from build123d import *

# Parameters (mm, degrees)
SKETCH1_R           = 1.5
BOSS_EXTRUDE1_DEPTH = 3
SKETCH2_W           = 6
SKETCH2_H           = 5
SKETCH2_H_2         = 2
BOSS_EXTRUDE2_DEPTH = 26
CUT_EXTRUDE1_REACH  = 34.939
SKETCH3_R           = 1.575
FILLET1_R           = 0.5


with BuildPart() as part:
    # Sketch1 → Boss-Extrude1 (new body)
    with BuildSketch(Plane(origin=(0, 0, 0), x_dir=(1, 0, 0), z_dir=(0, 1, 0))):
        Polygon((-10, 4.075667656), (10, 4.075667656), (10, -0.924332344), (3, -0.924332344), (3, -7.924332344), (-3, -7.924332344), (-3, -0.924332344), (-10, -0.924332344), align=None)
        with Locations(Location((7.5, 1.575667656, 0), (0, 0, 270))):
            Circle(SKETCH1_R, mode=Mode.SUBTRACT)
        with Locations(Location((-7.5, 1.575667656, 0), (0, 0, 270))):
            Circle(SKETCH1_R, mode=Mode.SUBTRACT)
    extrude(amount=BOSS_EXTRUDE1_DEPTH)

    # Sketch2 → Boss-Extrude2 (add)
    with BuildSketch(Plane(origin=(0, 3, 0), x_dir=(1, 0, 0), z_dir=(0, 1, 0))):
        with Locations((0, 1.575667656)):
            Rectangle(SKETCH2_W, SKETCH2_H)
        with Locations((0, -6.924332344)):
            Rectangle(SKETCH2_W, SKETCH2_H_2)
    extrude(amount=BOSS_EXTRUDE2_DEPTH)

    # Cut-Extrude1: up to this face of the body (flat: up to its plane)
    cut_extrude1_end = Plane(part.part.faces().sort_by_distance((0, 14.5, 7.924332344))[0])
    # Sketch3 → Cut-Extrude1 (cut, up to the picked face)
    with BuildSketch(Plane(origin=(0, 0, -4.075667656), x_dir=(-1, 0, 0), z_dir=(0, 0, -1)), mode=Mode.PRIVATE) as cut_extrude1_sk1:
        with Locations((0, 26.75)):
            Circle(SKETCH3_R)
    cut_extrude1_tool1 = split(extrude(cut_extrude1_sk1.sketch, amount=-CUT_EXTRUDE1_REACH, mode=Mode.PRIVATE), bisect_by=cut_extrude1_end, keep=Keep.BOTH, mode=Mode.PRIVATE)
    add(cut_extrude1_tool1.solids().sort_by(Axis((0, 26.75, -4.075668), (0, 0, 1)))[0], mode=Mode.SUBTRACT)

    # Fillet1
    fillet1_edges = [part.edges().sort_by_distance(p)[0] for p in [
        (1.575, 26.75, 0.924332344),
        (1.575, 26.75, 5.924332344),
        (1.575, 26.75, -4.075667656),
        (1.575, 26.75, 7.924332344),
    ]]
    fillet(fillet1_edges, radius=FILLET1_R)


solid = part.part
CAD build for the part. Positions are in the model's coordinates, mm. A direction names the side the tool comes from. Give positions to 0.01 mm unless a question says otherwise; leave off trailing zeros. Write each loop counter-clockwise with the first axis right and the second up, starting at its lowest first coordinate (ties: lowest second). Pieces come first, ordered by that corner, then holes. Notation, with made-up numbers: (25, -11) - (44, -11) arc R34 cw to (44, 24) - close; hole circle Ø5 at (-16, -23). An arc over 180 degrees is marked (long way). Answer as CSV lines item,"result".
Q1. Flat gauge pins, fed straight in: pin 1 Ø4 at (x, z) = (1, 3.5) entering from +Y; pin 2 Ø2.5 at (x, z) = (-7.5, -1.58) entering from +Y; pin 3 Ø2.5 at (x, y) = (5, 1) entering from +Z; pin 4 Ø3.5 at (x, y) = (0, 26.75) entering from +Z. Where does each tip first touch, or does it go through?
Result set:
pin 1,"y = 3"
pin 2,"through"
pin 3,"z = 0.92"
pin 4,"z = 7.8"
Q2. Pull direction Z, two halves, no side cores. Call faces 6 (the face through (6.036, 1.479, -1.901)), 7 (the face through (7, 1, 0.924)), 8 (the face through (3, 11, 7)): released by +Z, released by -Z, zero draft, split by the parting line, or undercut.
Result set:
face 6,"undercut"
face 7,"released by +Z"
face 8,"zero draft"
Q3. Band-saw the part on D-D (y = 12.75). Give the cut face in (x, z).
Result set:
outline,"(-3, -4.08) - (3, -4.08) - (3, 0.92) - (-3, 0.92) - close; (-3, 5.92) - (3, 5.92) - (3, 7.92) - (-3, 7.92) - close"
Q4. Band-saw the part on B-B (x = 0). Give the cut face in (y, z) (3 decimals).
Result set:
outline,"(0, -4.076) - (24.675, -4.076) arc R0.5 ccw to (25.175, -3.576) - (25.175, 0.424) arc R0.5 ccw to (24.675, 0.924) - (3, 0.924) - (3, 5.924) - (24.675, 5.924) arc R0.5 ccw to (25.175, 6.424) - (25.175, 7.424) arc R0.5 ccw to (24.675, 7.924) - (0, 7.924) - close; (28.325, -3.576) arc R0.5 ccw to (28.825, -4.076) - (29, -4.076) - (29, 0.924) - (28.825, 0.924) arc R0.5 ccw to (28.325, 0.424) - close; (28.325, 6.424) arc R0.5 ccw to (28.825, 5.924) - (29, 5.924) - (29, 7.924) - (28.825, 7.924) arc R0.5 ccw to (28.325, 7.424) - close"
Q5. Drill centre lines: line 1 (Y direction, x = 0, z = -1.15) (3 decimals); line 2 (X direction, y = 8.75, z = 7.5); line 3 (Y direction, x = 2, z = 4.75). Where is each one in solid material? Low to high. Write a range as from..to.
Result set:
line 1,"0..25.175, 28.325..29"
line 2,"-3..3"
line 3,"0..3"
Q6. Band-saw the part on A-A (x = 7.5). Give the cut face in (y, z), and give its area (3 significant figures).
Result set:
outline,"(0, -4.08) - (3, -4.08) - (3, -3.08) - (0, -3.08) - close; (0, -0.08) - (3, -0.08) - (3, 0.92) - (0, 0.92) - close"
area,"6.00 mm²"
Q7. Band-saw the part on C-C (y = 26.75). Give the cut face in (x, z) (3 decimals), and give its area (3 significant figures).
Result set:
outline,"(-3, -4.076) - (-2.075, -4.076) arc R0.5 ccw to (-1.575, -3.576) - (-1.575, 0.424) arc R0.5 ccw to (-2.075, 0.924) - (-3, 0.924) - close; (-3, 5.924) - (-2.075, 5.924) arc R0.5 ccw to (-1.575, 6.424) - (-1.575, 7.424) arc R0.5 ccw to (-2.075, 7.924) - (-3, 7.924) - close; (1.575, -3.576) arc R0.5 ccw to (2.075, -4.076) - (3, -4.076) - (3, 0.924) - (2.075, 0.924) arc R0.5 ccw to (1.575, 0.424) - close; (1.575, 6.424) arc R0.5 ccw to (2.075, 5.924) - (3, 5.924) - (3, 7.924) - (2.075, 7.924) arc R0.5 ccw to (1.575, 7.424) - close"
area,"19.5 mm²"
Q8. 3-axis set-ups, long thin cutter, end or side, ignore diameter. For faces 1 (the face through (0, 16, 5.924)), 2 (the face through (0, 11, -4.076)), 3 (the face through (5.8, 3, -1.6)), 4 (the face through (-3, 11, 7)), 5 (the face through (-3, 16, -2)): which of +Z, -Z, +X, -X, +Y, -Y reach the whole face in a straight line?
Result set:
face 1,"+X, -X, +Y"
face 2,"-Z, +X, -X, +Y, -Y"
face 3,"+Z, -Z, +X, +Y"
face 4,"+Z, -X, +Y, -Y"
face 5,"+Z, -Z, -X, +Y"
